from build123d import *

# Parameters (mm, degrees)
F0_W     = 135
F0_H     = 190
F1_DEPTH = 130
F2_R     = 15.186523
F3_DEPTH = 15
F2_W     = 95
F2_H     = 65
F4_DEPTH = 1
F5_W     = 30
F5_H     = 33
F6_DEPTH = 5


with BuildPart() as f1:
    # F0 (on Front) → F1 (new body, symmetric)
    with BuildSketch(Plane.XZ):
        Rectangle(F0_W, F0_H)
    extrude(amount=F1_DEPTH, both=True)

    # F2 (on face) → F3 (join)
    with BuildSketch(Plane.XZ.offset(130)):
        with Locations((37.5, -30)):
            Circle(F2_R)
    extrude(amount=F3_DEPTH)

    # F2 (on face) → F4 (join)
    with BuildSketch(Plane.XZ.offset(130)):
        with Locations((0, 52.5)):
            Rectangle(F2_W, F2_H)
    extrude(amount=F4_DEPTH)

    # F5 (on face) → F6 (join)
    with BuildSketch(Plane(origin=(0, 130, 0), x_dir=(-1, 0, 0), z_dir=(0, 1, 0))):
        with Locations((32.5, -51.5)):
            Rectangle(F5_W, F5_H)
    extrude(amount=F6_DEPTH)


solid = f1.part
Work out the finished part from the listing and answer in its coordinate system (mm). A direction names the side the tool comes from. Give positions to 0.01 mm unless a question says otherwise; leave off trailing zeros. Loops run counter-clockwise (first coordinate to the right, second up) from the corner with the lowest first, then second, coordinate; pieces in that order, holes last. Notation, with made-up numbers: (-34.75, 68.5) - (-9.75, 68.5) arc R14 ccw to (-9.75, 92.5) - close; hole circle Ø5 at (33.5, 24.25). An arc over 180 degrees is marked (long way). Answer in a Markdown table with one row per item. Add a question column.
Q1. The part is cut by section A-A (z = 61). Determine the outline of the cut face in (x, y).
Q2. Each of these flat-tipped pins is pushed along its axis until it touches: P1, Ø0.5, axis at y = -130.5, z = 68.5, coming from the +X side; P2, Ø1.5, axis at x = -28.5, y = 132, coming from the -Z side; P3, Ø4, axis at y = 133.5, z = -48, coming from the -X side. Where does it stop, or does it pass through?
Q3. A tool of negligible diameter and unlimited length cuts with its end or side. For faces 1 (the flat face through (-1, -131, 53)), 2 (the cylindrical face through (51.985, -137.395, -25.438)), 3 (the flat face through (-32, 135, -51)), from which of +Z, -Z, +X, -X, +Y, -Y can it reach the whole face along a straight path? Write none if from no direction.
Q4. Consider line 1 along Y through (x, z) = (10.5, -33.5); line 2 along Y through (x, z) = (8, 23.5). Determine where each line is inside the solid, lowest interval first.
Q5. The part is cut by section D-D (x = 37.5). Determine the outline of the cut face in (y, z), and give its area (3 significant figures).
Q6. The part is cut by section B-B (x = -37). Determine the outline of the cut face in (y, z), and give its area (3 significant figures).
Q7. The part is cut by section C-C (z = -30). Determine the outline of the cut face in (x, y), and give its area (3 significant figures).
Solution:
| question | item | result |
|---|---|---|
| 1 | outline | (-67.5, -130) - (-47.5, -130) - (-47.5, -131) - (47.5, -131) - (47.5, -130) - (67.5, -130) - (67.5, 130) - (-67.5, 130) - close |
| 2 | P1 | stops at x = 47.5 |
| 2 | P2 | stops at z = -68 |
| 2 | P3 | stops at x = -47.5 |
| 3 | face 1 | +Z, +X, -X, -Y |
| 3 | face 2 | -Y |
| 3 | face 3 | +Z, -Z, +X, -X, +Y |
| 4 | line 1 | y = -130 to 130 |
| 4 | line 2 | y = -131 to 130 |
| 5 | outline | (-145, -45.19) - (-130, -45.19) - (-130, -95) - (130, -95) - (130, 95) - (-130, 95) - (-130, 85) - (-131, 85) - (-131, 20) - (-130, 20) - (-130, -14.81) - (-145, -14.81) - close |
| 5 | area | 49,900 mm² |
| 6 | outline | (-131, 20) - (-130, 20) - (-130, -95) - (130, -95) - (130, -68) - (135, -68) - (135, -35) - (130, -35) - (130, 95) - (-130, 95) - (-130, 85) - (-131, 85) - close |
| 6 | area | 49,600 mm² |
| 7 | outline | (-67.5, -130) - (22.31, -130) - (22.31, -145) - (52.69, -145) - (52.69, -130) - (67.5, -130) - (67.5, 130) - (-67.5, 130) - close |
| 7 | area | 35,600 mm² |
